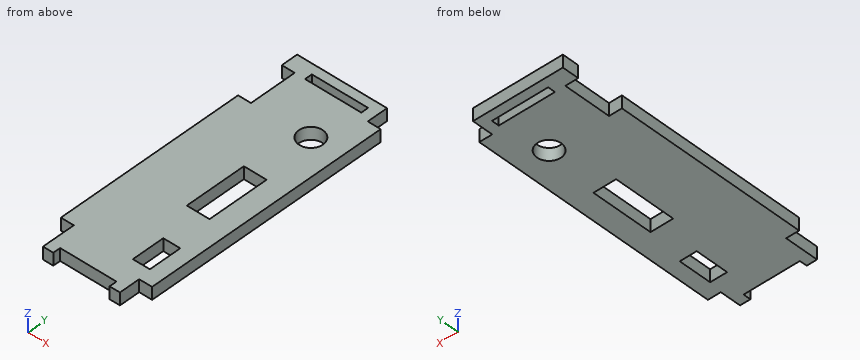
```python
from build123d import *

# Parameters (mm, degrees)
SKETCH1_W           = 4.1783
SKETCH1_H           = 8.0391
SKETCH1_W_2         = 5.588
SKETCH1_H_2         = 15.0876
SKETCH1_W_3         = 13.843
SKETCH1_H_3         = 1.8034
SKETCH1_R           = 2.96545
BOSS_EXTRUDE1_DEPTH = 3.048


with BuildPart() as part:
    # Sketch1 → Boss-Extrude1 (new body)
    with BuildSketch(Plane.XY):
        Polygon((3.175, 64.77), (3.175, 53.213), (0, 53.213), (0, 6.35), (3.175, 6.35), (3.175, -1.8034), (5.715, -1.8034), (5.715, 0), (19.558, 0), (19.558, -1.8034), (22.098, -1.8034), (22.098, 3.2766), (25.273, 3.2766), (25.273, 63.754), (22.098, 63.754), (22.098, 68.834), (0, 68.834), (0, 64.77), align=None)
        with Locations((19.52625, 10.64895)):
            Rectangle(SKETCH1_W, SKETCH1_H, mode=Mode.SUBTRACT)
        with Locations((17.1069, 31.8008)):
            Rectangle(SKETCH1_W_2, SKETCH1_H_2, mode=Mode.SUBTRACT)
        with Locations((12.6365, 65.6717)):
            Rectangle(SKETCH1_W_3, SKETCH1_H_3, mode=Mode.SUBTRACT)
        with Locations(Location((17.64665, 53.48605, 0), (0, 0, 180))):
            Circle(SKETCH1_R, mode=Mode.SUBTRACT)
    extrude(amount=BOSS_EXTRUDE1_DEPTH)


solid = part.part
```
Check sheet for the modelled part. Datum: model origin and axes. Units: mm. Round coordinates to 2 decimals unless told otherwise and drop trailing zeros. Loops run counter-clockwise (first coordinate to the right, second up) from the corner with the lowest first, then second, coordinate; pieces in that order, holes last. Notation, with made-up numbers: (10, -17.5) - (29, -17.5) arc R16 ccw to (29, 1.5) - close; hole circle Ø1 at (15, 39). An arc over 180 degrees is marked (long way). Answer as a JSON object with one key per item and string values. Group by question number.
Q1. Gauge pin test, flat ends, axial feed: P1, Ø9.5, axis at x = 17.65, y = 53.49, coming from the -Z side; P2, Ø0.9, axis at x = 23, z = 2, coming from the -Y side; P3, Ø0.9, axis at y = 60.5, z = 2, coming from the -X side (3 decimals); P4, Ø1.4, axis at y = -1, z = 1, coming from the +X side. Record the tip position at first contact, or that the pin passes through.
Q2. Sectioned sample at A-A, the plane x = 12. Enter the section's corners in (y, z).
Q3. Sectioned sample at D-D, the plane z = 1.95. Count the separate pieces of the cut face and the enclosed holes in it, plus the area to 3 significant figures.
Q4. Scan lines: line 1 along Y through (x, z) = (1, 2.85); line 2 along Y through (x, z) = (17.5, 1.3); line 3 along Y through (x, z) = (7, 1.3). Record each from-to range of solid material in increasing order. Write a range as [from, to].
Q5. Sectioned sample at C-C, the plane x = 16. Enter the section's corners in (y, z), plus the area to 3 significant figures.
Q6. Sectioned sample at B-B, the plane y = 38.5. Enter the section's corners in (x, z).
Solution:
{
 "1": {"P1": "stops at z = 0", "P2": "stops at y = 3.28", "P3": "stops at x = 3.175", "P4": "stops at x = 22.1"},
 "2": {"outline": "(0, 0) - (64.77, 0) - (64.77, 3.05) - (0, 3.05) - close; (66.57, 0) - (68.83, 0) - (68.83, 3.05) - (66.57, 3.05) - close"},
 "3": {"separate pieces": "1", "enclosed holes": "4", "area": "1,490 mm²"},
 "4": {"line 1": "y = [6.35, 53.21], [64.77, 68.83]", "line 2": "y = [0, 6.63], [14.67, 24.26], [39.34, 50.52], [56.45, 64.77], [66.57, 68.83]", "line 3": "y = [0, 64.77], [66.57, 68.83]"},
 "5": {"outline": "(0, 0) - (24.26, 0) - (24.26, 3.05) - (0, 3.05) - close; (39.34, 0) - (51.02, 0) - (51.02, 3.05) - (39.34, 3.05) - close; (55.95, 0) - (64.77, 0) - (64.77, 3.05) - (55.95, 3.05) - close; (66.57, 0) - (68.83, 0) - (68.83, 3.05) - (66.57, 3.05) - close", "area": "143 mm²"},
 "6": {"outline": "(0, 0) - (14.31, 0) - (14.31, 3.05) - (0, 3.05) - close; (19.9, 0) - (25.27, 0) - (25.27, 3.05) - (19.9, 3.05) - close"}
}
